Geometry: final body of the model. Coordinates: model frame, mm. A direction names the side the tool comes from. Round coordinates to 2 decimals unless told otherwise and drop trailing zeros. Loops run counter-clockwise (first coordinate to the right, second up) from the corner with the lowest first, then second, coordinate; pieces in that order, holes last. Notation, with made-up numbers: (69, -6) - (86, -6) arc R26 cw to (86, 29) - close; hole circle Ø8 at (-8, 35.5). An arc over 180 degrees is marked (long way). Answer as a JSON object with one key per item and string values. Group by question number.
Item 1: First-contact query: pin 1 (3 mm diameter, centred on x = -2, y = 2, fed in from +Z); pin 2 (4 mm diameter, centred on y = 4.5, z = 26, fed in from -X); pin 3 (1 mm diameter, centred on x = 8, z = 23, fed in from +Y). Flat tips, straight axial feed; report the tip coordinate or a pass-through.
Item 2: Section B-B (y = -0.75). Return the cut outline in (x, z).
Item 3: Reachability of faces 1 (the face through (-1.08, -4.88, -0.49)), 2 (the face through (-1.08, -4.88, 29.51)), 3 (the face through (-0.867, -3.905, 14.703)) from +Z, -Z, +X, -X, +Y, -Y: full face, straight path, thin tool, end or side. Return the list, or none.
Item 4: Line query: line 1 (Y direction, x = 0, z = 21.75); line 2 (Y direction, x = 0.5, z = 8); line 3 (Z direction, x = -7.25, y = -6.5). Output: solid intervals per line, ascending.
Item 5: Section D-D (y = 9). Return the cut outline in (x, z), plus the area to 3 significant figures.
Item 6: Section C-C (z = 26.5). Return the cut outline in (x, y), plus the area to 3 significant figures.
Item 7: Draft query along Y for faces 4 (the face through (-0.325, 8.536, 14.703)), 5 (the face through (6, -3, 29)), 6 (the face through (-5.994, 0.264, 29.493)). Return one class per face: released by +Y, released by -Y, zero draft, split by the parting line, or undercut.
Item 8: Section A-A (x = 0). Return the cut outline in (y, z), plus the area to 3 significant figures.
```python
from build123d import *

# Parameters (mm, degrees)
SKETCH1_R           = 13
SKETCH1_R_2         = 5
BOSS_EXTRUDE1_DEPTH = 29
SKETCH2_R           = 6
SKETCH2_R_2         = 5
BOSS_EXTRUDE2_DEPTH = 1
SKETCH3_R           = 1.5
CUT_EXTRUDE1_DEPTH  = 31
SKETCH4_R           = 5
SKETCH4_R_2         = 4
BOSS_EXTRUDE3_DEPTH = 29


with BuildPart() as part:
    # Sketch1 → Boss-Extrude1 (new body)
    with BuildSketch(Plane.XY):
        Circle(SKETCH1_R)
        Circle(SKETCH1_R_2, mode=Mode.SUBTRACT)
    extrude(amount=BOSS_EXTRUDE1_DEPTH)

    # Sketch2 → Boss-Extrude2 (add)
    with BuildSketch(Plane.XY.offset(29)):
        Circle(SKETCH2_R)
        Circle(SKETCH2_R_2, mode=Mode.SUBTRACT)
    boss_extrude2 = extrude(amount=BOSS_EXTRUDE2_DEPTH)

    # Mirror1: Boss-Extrude2 across plane
    add(boss_extrude2.mirror(Plane.XY.offset(14.5)))

    # Sketch3 → Cut-Extrude1 (cut, through all)
    with BuildSketch(Plane.XY.offset(29)):
        with Locations((0, 10)):
            Circle(SKETCH3_R)
        with Locations((8.660254038, -5)):
            Circle(SKETCH3_R)
        with Locations((-8.660254038, -5)):
            Circle(SKETCH3_R)
    extrude(amount=-CUT_EXTRUDE1_DEPTH, mode=Mode.SUBTRACT)

    # Sketch4 → Boss-Extrude3 (add)
    with BuildSketch(Plane.XY.offset(29)):
        Circle(SKETCH4_R)
        Circle(SKETCH4_R_2, mode=Mode.SUBTRACT)
    extrude(amount=-BOSS_EXTRUDE3_DEPTH)


solid = part.part
```
Values:
{
 "1": {"pin 1": "stops at z = 29", "pin 2": "stops at x = -12.76", "pin 3": "stops at y = 10.62"},
 "2": {"outline": "(-12.98, 0) - (-5.95, 0) - (-5.95, -1) - (-4.94, -1) - (-4.94, 0) - (-3.93, 0) - (-3.93, 29) - (-4.94, 29) - (-4.94, 30) - (-5.95, 30) - (-5.95, 29) - (-12.98, 29) - close; (3.93, 0) - (4.94, 0) - (4.94, -1) - (5.95, -1) - (5.95, 0) - (12.98, 0) - (12.98, 29) - (5.95, 29) - (5.95, 30) - (4.94, 30) - (4.94, 29) - (3.93, 29) - close"},
 "3": {"face 1": "-Z", "face 2": "+Z", "face 3": "+Z, -Z"},
 "4": {"line 1": "y = -13 to -4, 4 to 8.5, 11.5 to 13", "line 2": "y = -12.99 to -3.97, 3.97 to 8.59, 11.41 to 12.99", "line 3": "z = 0 to 29"},
 "5": {"outline": "(-9.38, 0) - (-1.12, 0) - (-1.12, 29) - (-9.38, 29) - close; (1.12, 0) - (9.38, 0) - (9.38, 29) - (1.12, 29) - close", "area": "479 mm^2"},
 "6": {"outline": "circle Ø26 at (0, 0); hole circle Ø3 at (-8.66, -5); hole circle Ø8 at (0, 0); hole circle Ø3 at (0, 10); hole circle Ø3 at (8.66, -5)", "area": "459 mm^2"},
 "7": {"face 4": "undercut", "face 5": "zero draft", "face 6": "split by the parting line"},
 "8": {"outline": "(-13, 0) - (-6, 0) - (-6, -1) - (-5, -1) - (-5, 0) - (-4, 0) - (-4, 29) - (-5, 29) - (-5, 30) - (-6, 30) - (-6, 29) - (-13, 29) - close; (4, 0) - (5, 0) - (5, -1) - (6, -1) - (6, 0) - (8.5, 0) - (8.5, 29) - (6, 29) - (6, 30) - (5, 30) - (5, 29) - (4, 29) - close; (11.5, 0) - (13, 0) - (13, 29) - (11.5, 29) - close", "area": "439 mm^2"}
}
